Part model, mm, in its own coordinate system. Face numbers are marked on the shaded views. Give positions to 0.01 mm unless a question says otherwise; leave off trailing zeros. Order: outer loops, then holes, each group sorted by start corner. A loop starts at its lowest first (then second) coordinate and runs counter-clockwise, first axis right, second up. Notation, with made-up numbers: (34.25, -27.5) -> (45.25, -27.5) arc R35 ccw to (45.25, 8.5) -> close; hole circle Ø9 at (59, 74.25). An arc over 180 degrees is marked (long way). Write item = value, one per line. Start each with the question number.
(1) Two-plate mould, pull along Z, no slides. Class the marked faces 1, 2, 3 and 4: pulls with the +Z half, pulls with the -Z half, needs draft (parallel to the pull), parting line crosses it, or undercut.
(2) Probe line 1 along Z through (x, y) = (0, 5.75); line 2 along X through (y, z) = (6.5, -34); line 3 along X through (y, z) = (9.5, -22). List the from-to ranges inside material, lowest first. Write a range as from..to.
(3) Saw through at B-B, the plane x = 49.52. List the corners of the cut face in (y, z), then the cut area to 3 significant figures.
(4) Saw through at D-D, the plane y = 6. State how many separate pieces and enclosed holes the cut face has, then the cut area to 3 significant figures.
(5) Saw through at C-C, the plane z = 0. List the corners of the cut face in (x, y).
(6) Saw through at A-A, the plane z = 49.52. List the corners of the cut face in (x, y).
(7) Flat gauge pins, fed straight in: pin 1 (2 mm diameter, centred on y = 2.5, z = -12, fed in from -X); pin 2 (11 mm diameter, centred on x = 2, z = 33.5, fed in from +Y); pin 3 (5 mm diameter, centred on x = 30, y = 5, fed in from +Z). Where does each tip first touch, or does it go through?
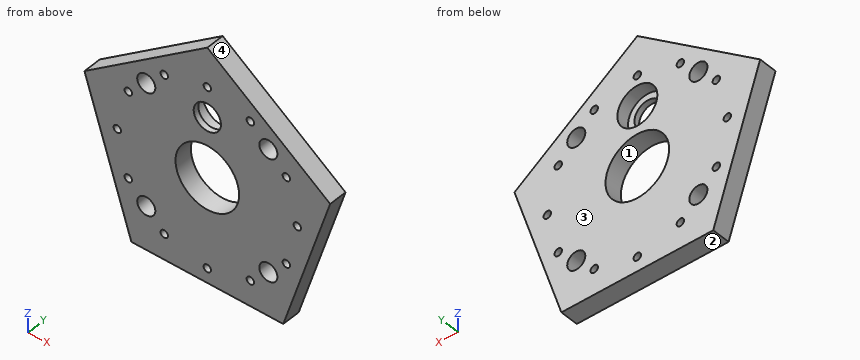
from build123d import *

# Parameters (mm, degrees)
BOSS_EXTRUDE1_DEPTH = 10
SKETCH2_R           = 11
CUT_EXTRUDE1_DEPTH  = 7
SKETCH3_R           = 7.5
CUT_EXTRUDE2_DEPTH  = 4
SKETCH5_R           = 4.975
SKETCH5_R_2         = 2.05
CUT_EXTRUDE4_DEPTH  = 11
SKETCH6_R           = 2.05
CUT_EXTRUDE5_DEPTH  = 11
CIRPATTERN1_COUNT   = 4
SKETCH7_R           = 17.5
CUT_EXTRUDE6_DEPTH  = 11


with BuildPart() as part:
    # Sketch1 → Boss-Extrude1 (new body)
    with BuildSketch(Plane(origin=(0, 0, 0), x_dir=(1, 0, 0), z_dir=(0, 1, 0))):
        Polygon((0, -71.073908706), (67.595304014, -21.963045647), (41.77619536, 57.5), (-41.77619536, 57.5), (-67.595304014, -21.963045647), align=None)
    extrude(amount=BOSS_EXTRUDE1_DEPTH)

    # Sketch2 → Cut-Extrude1 (cut)
    with BuildSketch(Plane(origin=(0, 10, 0), x_dir=(1, 0, 0), z_dir=(0, 1, 0))):
        with Locations((0, -33)):
            Circle(SKETCH2_R)
    extrude(amount=-CUT_EXTRUDE1_DEPTH, mode=Mode.SUBTRACT)

    # Sketch3 → Cut-Extrude2 (cut, through all)
    with BuildSketch(Plane(origin=(0, 3, 0), x_dir=(1, 0, 0), z_dir=(0, 1, 0))):
        with Locations((0, -33)):
            Circle(SKETCH3_R)
    extrude(amount=-CUT_EXTRUDE2_DEPTH, mode=Mode.SUBTRACT)

    # Sketch5 → Cut-Extrude4 (cut, through all)
    with BuildSketch(Plane(origin=(0, 10, 0), x_dir=(1, 0, 0), z_dir=(0, 1, 0))):
        with Locations((-33.587572106, -33.587572106)):
            Circle(SKETCH5_R)
        with Locations((-43.487067043, -23.68807717)):
            Circle(SKETCH5_R_2)
        with Locations((-23.68807717, -43.487067043)):
            Circle(SKETCH5_R_2)
    cut_extrude4 = extrude(amount=-CUT_EXTRUDE4_DEPTH, mode=Mode.SUBTRACT)

    # Sketch6 → Cut-Extrude5 (cut, through all)
    with BuildSketch(Plane(origin=(0, 10, 0), x_dir=(1, 0, 0), z_dir=(0, 1, 0))):
        with Locations((0, -49.52)):
            Circle(SKETCH6_R)
    cut_extrude5 = extrude(amount=-CUT_EXTRUDE5_DEPTH, mode=Mode.SUBTRACT)

    # CirPattern1: Cut-Extrude4, Cut-Extrude5 ×4 about axis
    cirpattern1_axis = Axis((0, 0, 0), (0, 1, 0))
    for i in range(1, CIRPATTERN1_COUNT):
        add(cut_extrude4.rotate(cirpattern1_axis, i * 360 / CIRPATTERN1_COUNT), mode=Mode.SUBTRACT)
        add(cut_extrude5.rotate(cirpattern1_axis, i * 360 / CIRPATTERN1_COUNT), mode=Mode.SUBTRACT)

    # Sketch7 → Cut-Extrude6 (cut, through all)
    with BuildSketch(Plane(origin=(0, 10, 0), x_dir=(1, 0, 0), z_dir=(0, 1, 0))):
        Circle(SKETCH7_R)
    extrude(amount=-CUT_EXTRUDE6_DEPTH, mode=Mode.SUBTRACT)


solid = part.part
Results list:
q1.face_1 = undercut
q1.face_2 = pulls with the -Z half
q1.face_3 = needs draft
q1.face_4 = pulls with the +Z half
q2.line_1 = -57.5..-51.57, -47.47..-17.5, 17.5..22, 44..47.47, 51.57..71.07
q2.line_2 = -49.41..-38.55, -28.63..28.63, 38.55..49.41
q2.line_3 = -53.31..-44.65, -42.32..42.32, 44.65..53.31
q3.outline = (0, -33.67) -> (10, -33.67) -> (10, -2.05) -> (0, -2.05) -> close; (0, 2.05) -> (10, 2.05) -> (10, 35.1) -> (0, 35.1) -> close
q3.area = 647 mm^2
q4.separate_pieces = 1
q4.enclosed_holes = 18
q4.area = 10,200 mm^2
q5.outline = (-60.46, 0) -> (-51.57, 0) -> (-51.57, 10) -> (-60.46, 10) -> close; (-47.47, 0) -> (-17.5, 0) -> (-17.5, 10) -> (-47.47, 10) -> close; (17.5, 0) -> (47.47, 0) -> (47.47, 10) -> (17.5, 10) -> close; (51.57, 0) -> (60.46, 0) -> (60.46, 10) -> (51.57, 10) -> close
q6.outline = (-29.67, 0) -> (-2.05, 0) -> (-2.05, 10) -> (-29.67, 10) -> close; (2.05, 0) -> (29.67, 0) -> (29.67, 10) -> (2.05, 10) -> close
q7.pin_1 = -56.88
q7.pin_2 = 3
q7.pin_3 = 51.09
